```python
from build123d import *

# Parameters (mm, degrees)
BOSS_EXTRU_1_DEPTH                                 = 3
D_GAGEMENT_61_D                                    = 4.3053
CHAMBRAGE_POUR_VIS_T_TE_RONDE_BOMB_E_M_D           = 3.1
CHAMBRAGE_POUR_VIS_T_TE_RONDE_BOMB_E_M_CBORE_D     = 6
CHAMBRAGE_POUR_VIS_T_TE_RONDE_BOMB_E_M_CBORE_DEPTH = 2.1
ESQUISSE7_W                                        = 5
ESQUISSE7_H                                        = 20
BOSS_EXTRU_2_DEPTH                                 = 6
ENL_V_MAT_EXTRU_1_REACH                            = 117.583
ESQUISSE8_W                                        = 2
ESQUISSE8_H                                        = 6
ENL_V_MAT_EXTRU_2_REACH                            = 83.526
ESQUISSE9_W                                        = 6
ESQUISSE9_H                                        = 2
ENL_V_MAT_EXTRU_3_REACH                            = 122.973
ESQUISSE10_W                                       = 2
ESQUISSE10_H                                       = 6
CONG_1_R                                           = 2
D_GAGEMENT_65_D                                    = 4.3053
D_GAGEMENT_64_D                                    = 4.3053


with BuildPart() as part:
    # Esquisse1 → Boss.-Extru.1 (new body)
    with BuildSketch(Plane.XY):
        Polygon((0, 0), (26.638249305, 0), (26.638249305, -109.993030409), (1.238249305, -109.993030409), (1.238249305, -33.176189805), (-23.361750695, -33.176189805), (-23.361750695, 0), align=None)
    extrude(amount=BOSS_EXTRU_1_DEPTH)

    # Dégagement #61 (through all)
    with Locations(Plane.XY.offset(3)):
        with Locations((21.47630139, -69.193030409), (7.67630139, -69.193030409), (7.617175732, -82.993030409), (21.538249305, -82.993030409)):
            Hole(D_GAGEMENT_61_D / 2)

    # Chambrage pour vis à tête ronde bombée M2.51 (through all)
    with Locations(Plane(origin=(0, 0, 0), x_dir=(-1, 0, 0), z_dir=(0, 0, -1))):
        with Locations((13.961750695, -23), (13.961750695, -11), (-10.038249305, -11), (-10.038249305, -23)):
            CounterBoreHole(CHAMBRAGE_POUR_VIS_T_TE_RONDE_BOMB_E_M_D / 2, CHAMBRAGE_POUR_VIS_T_TE_RONDE_BOMB_E_M_CBORE_D / 2, CHAMBRAGE_POUR_VIS_T_TE_RONDE_BOMB_E_M_CBORE_DEPTH)

    # Esquisse7 → Boss.-Extru.2 (add)
    with BuildSketch(Plane(origin=(0, 0, 0), x_dir=(-1, 0, 0), z_dir=(0, 0, -1))):
        Polygon((-11.638249305, -63.176189805), (-11.638249305, -33.176189805), (23.361750695, -33.176189805), (23.361750695, 0), (18.361750695, 0), (18.361750695, -28.176189805), (-16.638249305, -28.176189805), (-16.638249305, -63.176189805), align=None)
        with Locations((-14.138249305, -99.993030409)):
            Rectangle(ESQUISSE7_W, ESQUISSE7_H)
    extrude(amount=BOSS_EXTRU_2_DEPTH)

    # Esquisse8 → Enlèv. mat.-Extru.1 (cut, up to next)
    with BuildSketch(Plane.ZY.offset(-11.638249305), mode=Mode.PRIVATE) as enl_v_mat_extru_1_sk1:
        with Locations((-3, -49.176189805)):
            Rectangle(ESQUISSE8_W, ESQUISSE8_H)
    enl_v_mat_extru_1_tool1 = extrude(enl_v_mat_extru_1_sk1.sketch, amount=-ENL_V_MAT_EXTRU_1_REACH, mode=Mode.PRIVATE) & part.part
    add(enl_v_mat_extru_1_tool1.solids().sort_by_distance((11.638249, -49.17619, -3))[0], mode=Mode.SUBTRACT)

    # Esquisse9 → Enlèv. mat.-Extru.2 (cut, up to next)
    with BuildSketch(Plane.XZ.offset(33.176189805), mode=Mode.PRIVATE) as enl_v_mat_extru_2_sk1:
        with Locations((-3.361750695, -3)):
            Rectangle(ESQUISSE9_W, ESQUISSE9_H)
    enl_v_mat_extru_2_tool1 = extrude(enl_v_mat_extru_2_sk1.sketch, amount=-ENL_V_MAT_EXTRU_2_REACH, mode=Mode.PRIVATE) & part.part
    add(enl_v_mat_extru_2_tool1.solids().sort_by_distance((-3.361751, -33.17619, -3))[0], mode=Mode.SUBTRACT)

    # Esquisse10 → Enlèv. mat.-Extru.3 (cut, up to next)
    with BuildSketch(Plane.ZY.offset(23.361750695), mode=Mode.PRIVATE) as enl_v_mat_extru_3_sk1:
        with Locations((-3, -15.176189805)):
            Rectangle(ESQUISSE10_W, ESQUISSE10_H)
    enl_v_mat_extru_3_tool1 = extrude(enl_v_mat_extru_3_sk1.sketch, amount=-ENL_V_MAT_EXTRU_3_REACH, mode=Mode.PRIVATE) & part.part
    add(enl_v_mat_extru_3_tool1.solids().sort_by_distance((-23.361751, -15.17619, -3))[0], mode=Mode.SUBTRACT)

    # Congé1
    cong_1_edges = [part.edges().sort_by_distance(p)[0] for p in [
        (26.638249305, 0, 1.5),
        (26.638249305, -109.993030409, 1.5),
        (1.238249305, -109.993030409, 1.5),
        (1.238249305, -33.176189805, 1.5),
        (-23.361750695, -33.176189805, -1.5),
        (-23.361750695, 0, -1.5),
        (-18.361750695, -28.176189805, -3),
        (16.638249305, -28.176189805, -3),
        (11.638249305, -33.176189805, -3),
    ]]
    fillet(cong_1_edges, radius=CONG_1_R)

    # Dégagement #65 (through all)
    with Locations(Plane(origin=(0, 0, 0), x_dir=(-1, 0, 0), z_dir=(0, 0, -1))):
        with Locations((-23.638249305, -103.793030409), (-4.078249305, -103.793030409)):
            Hole(D_GAGEMENT_65_D / 2)

    # Dégagement #64 (through all)
    with Locations(Plane(origin=(0, 0, 0), x_dir=(-1, 0, 0), z_dir=(0, 0, -1))):
        with Locations((-23.798249305, -56.793030409), (-4.238249305, -56.793030409)):
            Hole(D_GAGEMENT_64_D / 2)


solid = part.part
```
Work out the finished part from the listing and answer in its coordinate system (mm). A direction names the side the tool comes from. Round coordinates to 2 decimals unless told otherwise and drop trailing zeros. Write each loop counter-clockwise with the first axis right and the second up, starting at its lowest first coordinate (ties: lowest second). Pieces come first, ordered by that corner, then holes. Notation, with made-up numbers: (31.25, 53.5) - (46.25, 53.5) arc R32 cw to (46.25, 87.5) - close; hole circle Ø2 at (-34, 61.25). An arc over 180 degrees is marked (long way). Return JSON: item names as keys, results as strings. Group by question number.
Q1. Each of these flat-tipped pins is pushed along its axis until it touches: pin 1 Ø7 at (x, y) = (4.24, -56.79) entering from -Z; pin 2 Ø0.6 at (x, z) = (-21.5, -3) entering from -Y; pin 3 Ø1.6 at (y, z) = (-31.5, -3) entering from +X. Where does it stop, or does it pass through?
Q2. The mould has two halves that part along X. Classify faces 1 (the flat face through (14, -100, -6)), 2 (the flat face through (-15.3, -24.3, 2.1)), 3 (the flat face through (-18.362, -12.9, -1.6)): released by +X, released by -X, zero draft, split by the parting line, or undercut.
Q3. Find the intervals of material crossed by L1, parallel to Y at x = -14, z = 2.5; L2, parallel to Y at x = 9, z = 1.25; L3, parallel to Y at x = 3.5, z = 2.5, in increasing order.
Q4. The part is cut by section C-C on x = -14.5. Write down the section's boundary in (y, z), then the cut area to 3 significant figures.
Q5. The part is cut by section B-B on x = -4. Write down the section's boundary in (y, z), then the cut area to 3 significant figures.
Q6. The part is cut by section A-A on y = -11. Write down the section's boundary in (x, z).
Q7. The part is cut by section D-D on y = -98.5. Write down the section's boundary in (x, z).
Q8. For faces 4 (the flat face through (14, -63.176, -3)), 5 (the flat face through (-3, -31, -2)), 6 (the flat face through (-21, -12.176, -3)), determine the directions among +Z, -Z, +X, -X, +Y, -Y from which every point of the face is accessible in a straight line to the end or side of a thin tool.
Solved:
{
 "1": {"pin 1": "z = 0", "pin 2": "y = -33.18", "pin 3": "x = 16.64"},
 "2": {"face 1": "zero draft", "face 2": "undercut", "face 3": "released by +X"},
 "3": {"L1": "-33.18 to -24.55, -21.45 to -12.55, -9.45 to 0", "L2": "-109.99 to -84.64, -81.34 to -70.89, -67.5 to -25.81, -20.19 to -13.81, -8.19 to 0", "L3": "-109.99 to -105.87, -101.72 to -58.82, -54.77 to 0"},
 "4": {"outline": "(-33.18, -6) - (-28.18, -6) - (-28.18, 0) - (-25.95, 0) - (-25.95, 2.1) - (-24.45, 2.1) - (-24.45, 3) - (-33.18, 3) - close; (-21.55, 2.1) - (-20.05, 2.1) - (-20.05, 0) - (-13.95, 0) - (-13.95, 2.1) - (-12.45, 2.1) - (-12.45, 3) - (-21.55, 3) - close; (-9.55, 2.1) - (-8.05, 2.1) - (-8.05, 0) - (0, 0) - (0, 3) - (-9.55, 3) - close", "area": "99.5 mm²"},
 "5": {"outline": "(-33.18, -6) - (-28.18, -6) - (-28.18, -4) - (-33.18, -4) - close; (-33.18, -2) - (-28.18, -2) - (-28.18, 0) - (0, 0) - (0, 3) - (-33.18, 3) - close", "area": "120 mm²"},
 "6": {"outline": "(-23.36, -6) - (-18.36, -6) - (-18.36, 0) - (-16.96, 0) - (-16.96, 2.1) - (-15.51, 2.1) - (-15.51, 3) - (-23.36, 3) - close; (-12.41, 2.1) - (-10.96, 2.1) - (-10.96, 0) - (7.04, 0) - (7.04, 2.1) - (8.49, 2.1) - (8.49, 3) - (-12.41, 3) - close; (11.59, 2.1) - (13.04, 2.1) - (13.04, 0) - (26.64, 0) - (26.64, 3) - (11.59, 3) - close"},
 "7": {"outline": "(1.24, 0) - (11.64, 0) - (11.64, -6) - (16.64, -6) - (16.64, 0) - (26.64, 0) - (26.64, 3) - (1.24, 3) - close"},
 "8": {"face 4": "-Z, +X, -X", "face 5": "+Y, -Y", "face 6": "+X, -X"}
}
